from build123d import *

# Parameters (mm, degrees)
PAD_DEPTH    = 7.5
SKETCH001_R  = 2.25
POCKET_DEPTH = 8
CHAMFER_SIZE = 1
FILLET_R     = 2
FILLET001_R  = 3
FILLET002_R  = 3
FILLET003_R  = 3


with BuildPart() as part:
    # Sketch → Pad (new body, symmetric)
    with BuildSketch(Plane.XZ):
        Polygon((0, 21.284523), (0, 91.284523), (8, 91.284523), (8, 66.284523), (31, 66.284523), (31, 78.284523), (39, 78.284523), (39, 53.435047), (8, 37.261134), (8, 22.261134), align=None)
        Polygon((8, 58.284523), (8, 46.284523), (31, 58.284523), align=None, mode=Mode.SUBTRACT)
    extrude(amount=PAD_DEPTH, both=True)

    # Sketch001 (on Face1 of Pad) → Pocket (cut)
    with BuildSketch(Plane(origin=(0, 0, 0), x_dir=(0, 0, -1), z_dir=(-1, 0, 0))):
        with Locations((-81.284523, 0)):
            Circle(SKETCH001_R)
        with Locations((-29.284523, 0)):
            Circle(SKETCH001_R)
    extrude(amount=-POCKET_DEPTH, mode=Mode.SUBTRACT)

    # Chamfer
    chamfer_edges = [part.edges().sort_by_distance(p)[0] for p in [
        (8, 0, 83.534523),
        (8, 0, 31.534523),
    ]]
    chamfer(chamfer_edges, length=CHAMFER_SIZE)

    # Fillet
    fillet_edges = [part.edges().sort_by_distance(p)[0] for p in [
        (4, -7.5, 91.284523),
        (4, 7.5, 91.284523),
    ]]
    fillet(fillet_edges, radius=FILLET_R)

    # Fillet001
    fillet001_edges = [part.edges().sort_by_distance(p)[0] for p in [
        (39, 0, 53.435047),
        (4, -7.5, 21.772828),
        (4, 7.5, 21.772828),
    ]]
    fillet(fillet001_edges, radius=FILLET001_R)

    # Fillet002
    fillet002_edges = [part.edges().sort_by_distance(p)[0] for p in [
        (35, -7.5, 78.284523),
        (35, 7.5, 78.284523),
        (8, 0, 37.261134),
    ]]
    fillet(fillet002_edges, radius=FILLET002_R)

    # Fillet003
    fillet003_edges = [part.edges().sort_by_distance(p)[0] for p in [
        (8, 0, 58.284523),
        (8, 0, 46.284523),
        (8, 0, 66.284523),
        (31, 0, 66.284523),
    ]]
    fillet(fillet003_edges, radius=FILLET003_R)


solid = part.part
Could you check a few things on this model? Use its own coordinates, in mm. A direction names the side the tool comes from. Coordinates: 2 decimals unless noted, no trailing zeros. Write each loop counter-clockwise with the first axis right and the second up, starting at its lowest first coordinate (ties: lowest second). Pieces come first, ordered by that corner, then holes. Notation, with made-up numbers: (31.25, 45) - (43.25, 45) arc R20 ccw to (43.25, 65) - close; hole circle Ø1 at (22, 87.5). An arc over 180 degrees is marked (long way). Put each result on its own line as item: value. Start each with the question number.
Q1. I'm going to push flat-ended pins straight in: P1, Ø2, axis at y = 1, z = 54, coming from the +X side; P2, Ø9, axis at x = 35.5, y = -1.5, coming from the +Z side; P3, Ø4.5, axis at y = -2, z = 83, coming from the +X side. Where does each tip first touch, or does it pass through?
Q2. I want a section at A-A on y = 0. Count the separate pieces of the cut face and the enclosed holes in it, plus the area to 3 significant figures.
Q3. Please list where these lines run through material, in increasing order: L1, parallel to X at y = -3.25, z = 73; L2, parallel to Z at x = 1.5, y = 0; L3, parallel to Z at x = 4.75, y = 0.
Q4. I want a section at B-B on x = 14.5. Write out the boundary of the cut face in (y, z), plus the area to 3 significant figures.
Q5. I want a section at D-D on x = 33.5. Write out the boundary of the cut face in (y, z), plus the area to 3 significant figures.
Q6. Thinking about a two-plate mould opening in Z: for faces 1 (the cylindrical face through (38.554, -0.105, 53.679)), 2 (the cylindrical face through (8.855, 0.105, 67.187)), 3 (the flat face through (21, 0, 58.285)), which applies, pulls with the +Z half, pulls with the -Z half, needs draft (parallel to the pull), parting line crosses it, or undercut?
Q7. Which directions (+Z, -Z, +X, -X, +Y, -Y) give clear straight access to the entire face, cutting with the end or side of a thin tool? Please do faces 4 (the flat face through (8, -3.4, 28.9)), 5 (the flat face through (35, 0, 78.285)), 6 (the cylindrical face through (9, 0, 49)), 7 (the cylindrical face through (35.056, -6.645, 77.382)), 8 (the cylindrical face through (35.056, 6.645, 77.382)).
Q8. I want a section at C-C on y = -6.25. Write out the boundary of the cut face in (x, z).
Checks:
1. P1: x = 38.99
1. P2: z = 78.28
1. P3: x = 8
2. separate pieces: 3
2. enclosed holes: 1
2. area: 1,100 mm²
3. L1: 0 to 8, 31 to 39
3. L2: 21.47 to 27.03, 31.53 to 79.03, 83.53 to 91.28
3. L3: 21.86 to 27.03, 31.53 to 79.03, 83.53 to 91.28
4. outline: (-7.5, 40.65) - (7.5, 40.65) - (7.5, 49.68) - (-7.5, 49.68) - close; (-7.5, 58.28) - (7.5, 58.28) - (7.5, 66.28) - (-7.5, 66.28) - close
4. area: 255 mm²
5. outline: (-7.5, 50.57) - (7.5, 50.57) - (7.5, 75.28) arc R3 ccw to (4.5, 78.28) - (-4.5, 78.28) arc R3 ccw to (-7.5, 75.28) - close
5. area: 412 mm²
6. face 1: pulls with the -Z half
6. face 2: pulls with the +Z half
6. face 3: undercut
7. face 4: -Z, +X, +Y, -Y
7. face 5: +Z, +X, +Y, -Y
7. face 6: +Y, -Y
7. face 7: +Z, +X, -Y
7. face 8: +Z, +X, +Y
8. outline: (0, 21.85) - (8, 22.83) - (8, 35.44) arc R3 cw to (9.61, 38.1) - (37.39, 52.59) arc R3 ccw to (39, 55.25) - (39, 77.72) - (31, 77.72) - (31, 69.28) arc R3 cw to (28, 66.28) - (11, 66.28) arc R3 cw to (8, 69.28) - (8, 91.14) - (0, 91.14) - close; hole (8, 51.23) arc R3 ccw to (12.39, 48.57) - (31, 58.28) - (11, 58.28) arc R3 ccw to (8, 55.28) - close
